The model under review builds one solid part; all positions refer to its coordinate system, in mm. Face numbers are marked on the shaded views. A direction names the side the tool comes from. Coordinates: 2 decimals unless noted, no trailing zeros. Write each loop counter-clockwise with the first axis right and the second up, starting at its lowest first coordinate (ties: lowest second). Pieces come first, ordered by that corner, then holes.
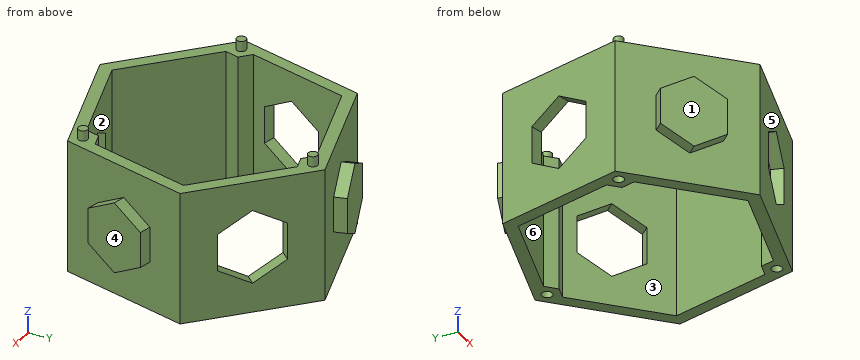
```python
from build123d import *

# Parameters (mm, degrees)
F1_DEPTH  = 32.332
F2_R      = 1.3
F3_DEPTH  = 3.5
F4_R      = 1.15
F5_DEPTH  = 2.5
F12_DEPTH = 3
F13_DEPTH = 3
F14_DEPTH = 3
F15_DEPTH = 3
F16_DEPTH = 3
F17_DEPTH = 3


# Not quite as in the source:
# - a feature names something its author has since deleted; it is built from what else it names


with BuildPart() as f1:
    # F0 (on Top) → F1 (new body)
    with BuildSketch(Plane.XY):
        Polygon((-7.7747095404, -31.3829129447), (23.2910450847, -22.4245524414), (31.0657546251, 8.9583605033), (7.7747095404, 31.3829129447), (-23.2910450847, 22.4245524414), (-31.0657546251, -8.9583605033), align=None)
        Polygon((21.6285805621, -16.6594668643), (20.7955759684, -20.0219218227), (17.4671022586, -20.9817461623), (-6.9417049468, -28.0204579863), (-25.241811799, -10.4011667824), (-27.7372809153, -7.9985361637), (-26.9042763216, -4.6360812053), (-20.7955759684, 20.0219218227), (3.613231237, 27.0606336467), (6.9417049468, 28.0204579863), (9.437174063, 25.6178273676), (27.7372809153, 7.9985361637), align=None, mode=Mode.SUBTRACT)
        Polygon((-27.7372809153, -7.9985361637), (-25.241811799, -10.4011667824), (-24.4088072054, -7.038711824), (-26.9042763216, -4.6360812053), align=None)
        Polygon((6.1087003532, 24.658003028), (9.437174063, 25.6178273676), (6.9417049468, 28.0204579863), (3.613231237, 27.0606336467), align=None)
        Polygon((17.4671022586, -20.9817461623), (20.7955759684, -20.0219218227), (21.6285805621, -16.6594668643), (18.3001068522, -17.619291204), align=None)
    extrude(amount=F1_DEPTH)

    # F2 (on face) → F3 (cut)
    with BuildSketch(Plane(origin=(0, 0, 0), x_dir=(1, 0, 0), z_dir=(0, 0, -1))):
        with Locations((20.7955759684, 20.0219218227)):
            Circle(F2_R)
        with Locations((6.9417049468, -28.0204579863)):
            Circle(F2_R)
        with Locations((-27.7372809153, 7.9985361637)):
            Circle(F2_R)
    extrude(amount=-F3_DEPTH, mode=Mode.SUBTRACT)

    # F4 (on face) → F5 (join)
    with BuildSketch(Plane.XY.offset(32.332)):
        with Locations((6.9417049468, 28.0204579863)):
            Circle(F4_R)
        with Locations((20.7955759684, -20.0219218227)):
            Circle(F4_R)
        with Locations((-27.7372809153, -7.9985361637)):
            Circle(F4_R)
    extrude(amount=F5_DEPTH)

    # F9 (on face) → F12 (join)
    with BuildSketch(Plane(origin=(27.1783998549, -6.7330959691, 0), x_dir=(0.2404677132, 0.9706571377, 0), z_dir=(0.9706571377, -0.2404677132, 0))):
        Polygon((-7.5, 20.4961270189), (-7.5, 11.8358729811), (0, 7.5057459622), (7.5, 11.8358729811), (7.5, 20.4961270189), (0, 24.8262540378), align=None)
    extrude(amount=F12_DEPTH)

    # F7 (on face) → F13 (join)
    with BuildSketch(Plane(origin=(-7.7581677721, 26.9037326931, 0), x_dir=(-0.9608475962, -0.2770774204, 0), z_dir=(-0.2770774204, 0.9608475962, 0))):
        Polygon((-7.5, 20.4961270189), (-7.5, 11.8358729811), (0, 7.5057459622), (7.5, 11.8358729811), (7.5, 20.4961270189), (0, 24.8262540378), align=None)
    extrude(amount=F13_DEPTH)

    # F11 (on face) → F14 (join)
    with BuildSketch(Plane(origin=(-19.4202320828, -20.170636724, 0), x_dir=(0.720379883, -0.6935797172, 0), z_dir=(-0.6935797172, -0.720379883, 0))):
        Polygon((-7.0119504524, 20.4961270189), (-7.0119504524, 11.8358729811), (0.4880495476, 7.5057459622), (7.9880495476, 11.8358729811), (7.9880495476, 20.4961270189), (0.4880495476, 24.8262540378), align=None)
    extrude(amount=F14_DEPTH)

    # F10 (on face) → F15 (cut, through all)
    with BuildSketch(Plane(origin=(7.7581677721, -26.9037326931, 0), x_dir=(0.9608475962, 0.2770774204, 0), z_dir=(0.2770774204, -0.9608475962, 0))):
        Polygon((-7.8, 20.6693320997), (-7.8, 11.6626679003), (0, 7.1593358006), (7.8, 11.6626679003), (7.8, 20.6693320997), (0, 25.1726641994), align=None)
    extrude(amount=-F15_DEPTH, mode=Mode.SUBTRACT)

    # F6 (on face) → F16 (cut, through all)
    with BuildSketch(Plane(origin=(-27.1783998549, 6.7330959691, 0), x_dir=(-0.2404677132, -0.9706571377, 0), z_dir=(-0.9706571377, 0.2404677132, 0))):
        Polygon((-7.8, 20.6693320997), (-7.8, 11.6626679003), (0, 7.1593358006), (7.8, 11.6626679003), (7.8, 20.6693320997), (0, 25.1726641994), align=None)
    extrude(amount=-F16_DEPTH, mode=Mode.SUBTRACT)

    # F8 (on face) → F17 (cut, through all)
    with BuildSketch(Plane(origin=(19.4202320828, 20.170636724, 0), x_dir=(-0.720379883, 0.6935797172, 0), z_dir=(0.6935797172, 0.720379883, 0))):
        Polygon((-7.8, 20.6693320997), (-7.8, 11.6626679003), (0, 7.1593358006), (7.8, 11.6626679003), (7.8, 20.6693320997), (0, 25.1726641994), align=None)
    extrude(amount=-F17_DEPTH, mode=Mode.SUBTRACT)


solid = f1.part
```
Item 1: Take a section at D-D, the plane x = 4.5. Write out the cut boundary in (y, z), plus the area to 3 significant figures.
Solved:
outline: (-27.84, 0) - (-24.72, 0) - (-24.72, 8.62) - (-27.84, 9.12) - close; (-27.84, 23.21) - (-24.72, 23.71) - (-24.72, 32.33) - (-27.84, 32.33) - close; (26.21, 0) - (30.44, 0) - (30.44, 32.33) - (26.21, 32.33) - close
area: 192 mm2
Item 2: Mouldability with a two-part tool opening along X and no side actions: class the marked faces 1, 2, 3 and 4 as pulls with the +X half, pulls with the -X half, needs draft (parallel to the pull), parting line crosses it, or undercut.
Solved:
face 1: pulls with the -X half
face 2: undercut
face 3: undercut
face 4: pulls with the +X half
Item 3: Take a section at C-C, the plane x = -3. Write out the cut boundary in (y, z).
Solved:
outline: (-30.01, 0) - (-26.88, 0) - (-26.88, 32.33) - (-30.01, 32.33) - close; (25.15, 0) - (28.28, 0) - (28.28, 10.36) - (31.4, 10.86) - (31.4, 21.47) - (28.28, 21.97) - (28.28, 32.33) - (25.15, 32.33) - close
Item 4: Machinability: for the marked faces 5 and 6, which of the approach directions +Z, -Z, +X, -X, +Y, -Y give a long, thin tool a straight path to every point of the face, cutting with its end or side? Answer none if there is none.
Solved:
face 5: +Z, -Z, +X, -Y
face 6: +Z, -Z
Item 5: Take a section at B-B, the plane y = 4. Write out the cut boundary in (x, z) (3 decimals).
Solved:
outline: (-27.855, 0) - (-24.765, 0) - (-24.765, 8.356) - (-27.855, 8.785) - close; (-27.855, 23.547) - (-24.765, 23.976) - (-24.765, 32.332) - (-27.855, 32.332) - close; (26.747, 0) - (29.837, 0) - (29.837, 32.332) - (26.747, 32.332) - close
Item 6: To check wall thickness, follow line 1 along Z through (x, y) = (-9.5, -26); line 2 along Y through (x, z) = (-19.5, 31.5); line 3 along X through (y, z) = (-15, 29). State the ranges of each line that lie inside material, in increasing order.
Solved:
line 1: z = 0 to 32.33
line 2: y = -20.09 to -15.93, 20.4 to 23.52
line 3: x = -24.79 to -20.47, 22.04 to 25.13
Item 7: For pin 1 (4 mm diameter, centred on x = 19.5, z = 13.5, fed in from -Y); pin 2 (1.3 mm diameter, centred on x = 6.5, y = 28, fed in from -Z); pin 3 (6 mm diameter, centred on x = -13, y = 19.5, fed in from +Z), all flat-tipped, find the tip position at first contact; note any pin that passes through.
Solved:
pin 1: stops at y = -24.09
pin 2: stops at z = 3.5
pin 3: stops at z = 32.33
Item 8: Take a section at A-A, the plane z = 5. Write out the cut boundary in (x, y).
Solved:
outline: (-31.07, -8.96) - (-7.77, -31.38) - (23.29, -22.42) - (31.07, 8.96) - (7.77, 31.38) - (-23.29, 22.42) - close; hole (-26.9, -4.64) - (-24.41, -7.04) - (-25.24, -10.4) - (-6.94, -28.02) - (17.47, -20.98) - (18.3, -17.62) - (21.63, -16.66) - (27.74, 8) - (9.44, 25.62) - (6.11, 24.66) - (3.61, 27.06) - (-20.8, 20.02) - close
